from build123d import *

# Parameters (mm, degrees)
SKETCH1_R           = 2.5796875
BOSS_EXTRUDE1_DEPTH = 1.5875


with BuildPart() as part:
    # Sketch1 → Boss-Extrude1 (new body, symmetric)
    with BuildSketch(Plane(origin=(0, 0, 0), x_dir=(1, 0, 0), z_dir=(0, 1, 0))):
        Polygon((25.4, -4.7879), (25.4, -12.7), (-25.4, -12.7), (-25.4, -4.7879), (-28.575, -4.7879), (-28.575, 4.7879), (-25.4, 4.7879), (-25.4, 12.7), (25.4, 12.7), (25.4, 4.7879), (28.575, 4.7879), (28.575, -4.7879), align=None)
        Circle(SKETCH1_R, mode=Mode.SUBTRACT)
    extrude(amount=BOSS_EXTRUDE1_DEPTH, both=True)


solid = part.part
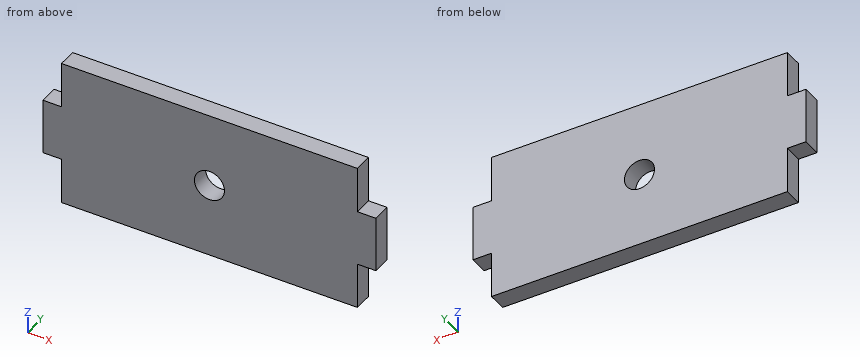
Geometry: final body of the model. Coordinates: model frame, mm. Give positions to 0.01 mm unless a question says otherwise; leave off trailing zeros. Write each loop counter-clockwise with the first axis right and the second up, starting at its lowest first coordinate (ties: lowest second). Pieces come first, ordered by that corner, then holes. Notation, with made-up numbers: (34.5, 60.5) - (51.5, 60.5) arc R24 ccw to (51.5, 89.5) - close; hole circle Ø9 at (87, 78.5). An arc over 180 degrees is marked (long way). Return JSON: item names as keys, results as strings. Group by question number.
1) First-contact query: P1, Ø4, axis at x = 0, z = 0, coming from the +Y side; P2, Ø1, axis at y = 0.5, z = 7, coming from the +X side; P3, Ø1, axis at y = 0.5, z = -9.5, coming from the -X side; P4, Ø1, axis at x = 27.5, y = 0, coming from the +Z side. Flat tips, straight axial feed; report the tip coordinate or a pass-through.
2) Section B-B on y = 0.6. Return the cut outline in (x, z) (3 decimals).
3) Section C-C on x = 0. Return the cut outline in (y, z), plus the area to 3 significant figures.
4) Section A-A on z = 0. Return the cut outline in (x, y) (1 decimal).
5) Line query: line 1 (X direction, y = -0.4, z = 0) (3 decimals); line 2 (Z direction, x = 0, y = -0.85); line 3 (X direction, y = 0.6, z = -1.25) (3 decimals). Output: solid intervals per line, ascending.
6) Section D-D on z = 10.5. Return the cut outline in (x, y), plus the area to 3 significant figures.
Filled in:
{
 "1": {"P1": "passes through", "P2": "stops at x = 25.4", "P3": "stops at x = -25.4", "P4": "stops at z = 4.79"},
 "2": {"outline": "(-28.575, -4.788) - (-25.4, -4.788) - (-25.4, -12.7) - (25.4, -12.7) - (25.4, -4.788) - (28.575, -4.788) - (28.575, 4.788) - (25.4, 4.788) - (25.4, 12.7) - (-25.4, 12.7) - (-25.4, 4.788) - (-28.575, 4.788) - close; hole circle Ø5.159 at (0, 0)"},
 "3": {"outline": "(-1.59, -12.7) - (1.59, -12.7) - (1.59, -2.58) - (-1.59, -2.58) - close; (-1.59, 2.58) - (1.59, 2.58) - (1.59, 12.7) - (-1.59, 12.7) - close", "area": "64.3 mm^2"},
 "4": {"outline": "(-28.6, -1.6) - (-2.6, -1.6) - (-2.6, 1.6) - (-28.6, 1.6) - close; (2.6, -1.6) - (28.6, -1.6) - (28.6, 1.6) - (2.6, 1.6) - close"},
 "5": {"line 1": "x = -28.575 to -2.58, 2.58 to 28.575", "line 2": "z = -12.7 to -2.58, 2.58 to 12.7", "line 3": "x = -28.575 to -2.257, 2.257 to 28.575"},
 "6": {"outline": "(-25.4, -1.59) - (25.4, -1.59) - (25.4, 1.59) - (-25.4, 1.59) - close", "area": "161 mm^2"}
}
